Here's the drawing with two shaded views (mm, measured from the low corner). I have some questions. Give positions to 0.01 mm unless a question says otherwise; leave off trailing zeros. Write each loop counter-clockwise with the first axis right and the second up, starting at its lowest first coordinate (ties: lowest second). Pieces come first, ordered by that corner, then holes. Notation, with made-up numbers: (20, 71.5) - (61, 71.5) arc R7 ccw to (61, 80.5) - close; hole circle Ø7 at (1, 29.25). An arc over 180 degrees is marked (long way). Answer as CSV lines item,"result". Start each with the question number.
Q1. If I drill on line 1 along Z through (x, y) = (7.5, 3); line 2 along X through (y, z) = (10, 35.5), over which ranges is the centre line in solid material (lowest first)?
Q2. Imagine slicing it at A-A on x = 3.5. List the corners of the cut face in (y, z) for me, and give its area (3 significant figures).
Q3. Imagine slicing it at B-B on y = 22. List the corners of the cut face in (x, z) for me.
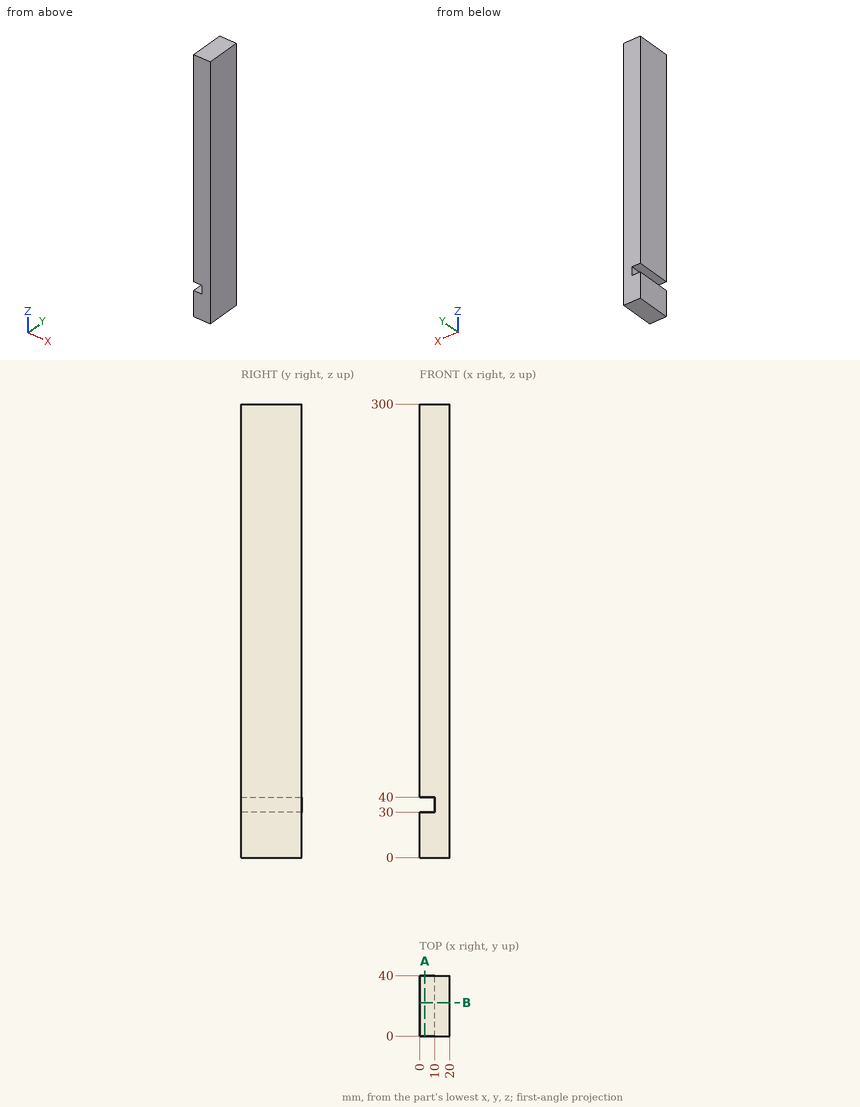
Conclusion:
1,line 1,"0 to 30, 40 to 300"
1,line 2,"10 to 20"
2,outline,"(0, 0) - (40, 0) - (40, 30) - (0, 30) - close; (0, 40) - (40, 40) - (40, 300) - (0, 300) - close"
2,area,"11,600 mm^2"
3,outline,"(0, 0) - (20, 0) - (20, 300) - (0, 300) - (0, 40) - (10, 40) - (10, 30) - (0, 30) - close"
